from build123d import *

# Parameters (mm, degrees)
F1_DEPTH = 9


with BuildPart() as f1:
    # F0 (on Top) → F1 (new body)
    with BuildSketch(Plane.XY):
        with BuildLine():
            ThreePointArc((0, -2.9), (-2.9, 0), (0, 2.9))
            Line((0, 2.9), (4, 2.9))
            ThreePointArc((4, 2.9), (4.353553, 3.046447), (4.5, 3.4))
            Line((4.5, 3.4), (4.5, 4))
            ThreePointArc((4.5, 4), (4.353553, 4.353553), (4, 4.5))
            Line((4, 4.5), (0, 4.5))
            ThreePointArc((0, 4.5), (-2.806243, 3.517812), (-4.387482, 1))
            Line((-4.387482, 1), (-35, 1))
            ThreePointArc((-35, 1), (-36, 0), (-35, -1))
            Line((-35, -1), (-4.387482, -1))
            ThreePointArc((-4.387482, -1), (-2.806243, -3.517812), (0, -4.5))
            Line((0, -4.5), (4, -4.5))
            ThreePointArc((4, -4.5), (4.353553, -4.353553), (4.5, -4))
            Line((4.5, -4), (4.5, -3.4))
            ThreePointArc((4.5, -3.4), (4.353553, -3.046447), (4, -2.9))
            Line((4, -2.9), (0, -2.9))
        make_face()
    extrude(amount=F1_DEPTH)


solid = f1.part
Verification items for the finished model (mm, model axes). A direction names the side the tool comes from. Give positions to 0.01 mm unless a question says otherwise; leave off trailing zeros. Write each loop counter-clockwise with the first axis right and the second up, starting at its lowest first coordinate (ties: lowest second). Pieces come first, ordered by that corner, then holes. Notation, with made-up numbers: M 39,27 L 66,27 A24 ccw 66,60 Z; hole C -24.75,37 d1. An arc over 180 degrees is marked long. Put each result on its own line as item: value. Start each with the question number.
1. Go/stop test with flat-tipped pins: pin 1 Ø2 at (y, z) = (-1.5, 7.5) entering from +X; pin 2 Ø3 at (y, z) = (-0.5, 3) entering from +X; pin 3 Ø5 at (y, z) = (3, 3) entering from -X; pin 4 Ø3 at (x, z) = (-1.5, 4) entering from -Y. Record where each tip stops, or that it passes through.
2. Section check A-A (z = 5). Record the cut outline in (x, y).
3. Scan lines: line 1 along Y through (x, z) = (2.5, 8.5); line 2 along Y through (x, z) = (-4.5, 2.5); line 3 along X through (y, z) = (0, 6.75). Record each from-to range of solid material in increasing order. Write a range as [from, to].
4. Section check B-B (y = 0). Record the cut outline in (x, z), and give its area (3 significant figures).
5. Section check C-C (x = -14.5). Record the cut outline in (y, z).
6. Set-up check for faces 1 (the face through (-19, 1, 4)), 2 (the face through (2, -2.9, 4)), 3 (the face through (-20, -1, 4)): record each of +Z, -Z, +X, -X, +Y, -Y from which the full face is reachable in a straight line by a thin tool's end or side.
7. Draft check along Y on faces 4 (the face through (-2.84, -3.49, 4.44)), 5 (the face through (2, 2.9, 4)), 6 (the face through (-2.773, 3.544, 4.437)). Enter one of: +Y half, -Y half, draft (parallel to the pull), parting line (faces both ways), or undercut.
Answer list:
1. pin 1: x = -1.47
1. pin 2: x = -2.1
1. pin 3: x = -35.87
1. pin 4: y = -4.5
2. outline: M -35,-1 L -4.39,-1 A4.5 ccw 0,-4.5 L 4,-4.5 A0.5 ccw 4.5,-4 L 4.5,-3.4 A0.5 ccw 4,-2.9 L 0,-2.9 A2.9 cw 0,2.9 L 4,2.9 A0.5 ccw 4.5,3.4 L 4.5,4 A0.5 ccw 4,4.5 L 0,4.5 A4.5 ccw -4.39,1 L -35,1 A1 ccw Z
3. line 1: [-4.5, -2.9], [2.9, 4.5]
3. line 2: [-1, 1]
3. line 3: [-36, -2.9]
4. outline: M -36,0 L -2.9,0 L -2.9,9 L -36,9 Z
4. area: 298 mm2
5. outline: M -1,0 L 1,0 L 1,9 L -1,9 Z
6. face 1: +Z, -Z, -X, +Y
6. face 2: +Z, -Z, +X
6. face 3: +Z, -Z, -X, -Y
7. face 4: -Y half
7. face 5: undercut
7. face 6: +Y half
